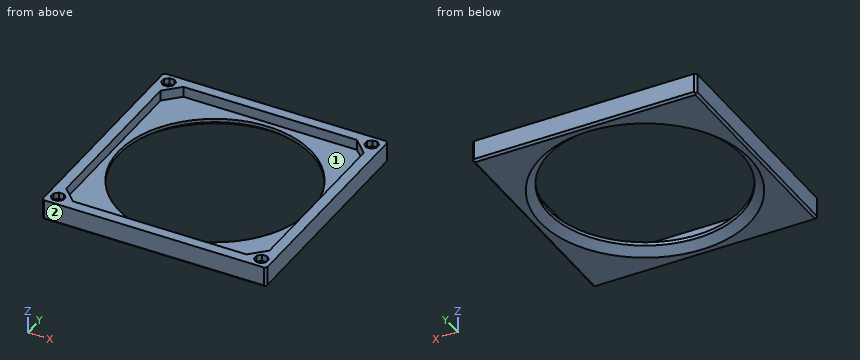
```python
from build123d import *

# Parameters (mm, degrees)
SKETCH1_LARGER_DIA_W    = 106
SKETCH1_LARGER_DIA_H    = 106
BOSS_EXTRUDE1_DEPTH     = 5
SKETCH5_SMALLER_DIA_W   = 106
SKETCH5_SMALLER_DIA_H   = 106
SKETCH5_SMALLER_DIA_R   = 45.5
BOSS_EXTRUDE2_DEPTH     = 5
CUT_EXTRUDE1_DEPTH      = 3
CHAMFER1_SIZE           = 4
CHAMFER1_SIZE2          = 3.356398525
CHAMFER2_SIZE           = 1
CHAMFER3_SIZE           = 1
CUT_EXTRUDE2_DEPTH      = 10
CUT_EXTRUDE2_DEPTH_BACK = 2
SKETCH3_HOLES_R         = 1.6


with BuildPart() as part:
    # Sketch1 larger dia → Boss-Extrude1 (new body)
    with BuildSketch(Plane.XY):
        Rectangle(SKETCH1_LARGER_DIA_W, SKETCH1_LARGER_DIA_H)
        Polygon((-41, 48), (41, 48), (48, 41), (48, -41), (41, -48), (-41, -48), (-48, -41), (-48, 41), align=None, mode=Mode.SUBTRACT)
    extrude(amount=BOSS_EXTRUDE1_DEPTH)

    # Sketch5 smaller dia → Boss-Extrude2 (add)
    with BuildSketch(Plane(origin=(0, 0, 0), x_dir=(-1, 0, 0), z_dir=(0, 0, -1))):
        Rectangle(SKETCH5_SMALLER_DIA_W, SKETCH5_SMALLER_DIA_H)
        Circle(SKETCH5_SMALLER_DIA_R, mode=Mode.SUBTRACT)
    extrude(amount=BOSS_EXTRUDE2_DEPTH)

    # Sketch1 → Cut-Extrude1 (cut)
    with BuildSketch(Plane.XY.offset(5)):
        Polygon((-45.1, 46.798780669), (-45.1, 49.201219331), (-46.798780669, 50.9), (-49.201219331, 50.9), (-50.9, 49.201219331), (-50.9, 46.798780669), (-49.201219331, 45.1), (-46.798780669, 45.1), align=None)
        Polygon((-46.798780669, -45.1), (-45.1, -46.798780669), (-45.1, -49.201219331), (-46.798780669, -50.9), (-49.201219331, -50.9), (-50.9, -49.201219331), (-50.9, -46.798780669), (-49.201219331, -45.1), align=None)
        Polygon((46.798780669, 45.1), (45.1, 46.798780669), (45.1, 49.201219331), (46.798780669, 50.9), (49.201219331, 50.9), (50.9, 49.201219331), (50.9, 46.798780669), (49.201219331, 45.1), align=None)
        Polygon((45.1, -46.798780669), (45.1, -49.201219331), (46.798780669, -50.9), (49.201219331, -50.9), (50.9, -49.201219331), (50.9, -46.798780669), (49.201219331, -45.1), (46.798780669, -45.1), align=None)
    extrude(amount=-CUT_EXTRUDE1_DEPTH, mode=Mode.SUBTRACT)

    # Chamfer1
    chamfer1_edges = [part.edges().sort_by_distance(p)[0] for p in [
        (45.5, 0, -5),
    ]]
    chamfer1_side = [part.faces().sort_by_distance(p)[0] for p in [
        (0, 51.500933624, -5),
    ]]
    chamfer(chamfer1_edges, length=CHAMFER1_SIZE, length2=CHAMFER1_SIZE2, reference=chamfer1_side[0])

    # Chamfer2
    chamfer2_edges = [part.edges().sort_by_distance(p)[0] for p in [
        (53, 0, -5),
        (0, -53, -5),
        (-53, 0, -5),
        (0, 53, -5),
    ]]
    chamfer(chamfer2_edges, length=CHAMFER2_SIZE)

    # Chamfer3
    chamfer3_edges = [part.edges().sort_by_distance(p)[0] for p in [
        (-53, 53, 0.5),
        (53, 53, 0.5),
        (53, -53, 0.5),
        (-53, -53, 0.5),
    ]]
    chamfer(chamfer3_edges, length=CHAMFER3_SIZE)

    # Sketch3 holes → Cut-Extrude2 (cut, two sides: drawn at the far end of the back side and taken through both)
    with BuildSketch(Plane.XY.offset(-CUT_EXTRUDE2_DEPTH_BACK)):
        with Locations((-48, 48)):
            Circle(SKETCH3_HOLES_R)
        with Locations(Location((48, 48, 0), (0, 0, 180))):
            Circle(SKETCH3_HOLES_R)
        with Locations(Location((-48, -48, 0), (0, 0, 180))):
            Circle(SKETCH3_HOLES_R)
        with Locations((48, -48)):
            Circle(SKETCH3_HOLES_R)
    extrude(amount=CUT_EXTRUDE2_DEPTH + CUT_EXTRUDE2_DEPTH_BACK, mode=Mode.SUBTRACT)


solid = part.part
```
Verification items for the finished model (mm, model axes). Face numbers are marked on the shaded views. Give positions to 0.01 mm unless a question says otherwise; leave off trailing zeros. Order: outer loops, then holes, each group sorted by start corner. A loop starts at its lowest first (then second) coordinate and runs counter-clockwise, first axis right, second up. Notation, with made-up numbers: (-13, -17.5) -> (5, -17.5) arc R15 ccw to (5, -12.5) -> close; hole circle Ø11 at (-38.5, -29). An arc over 180 degrees is marked (long way). One line per item, written item: value.
(1) Scan lines: line 1 along X through (y, z) = (-48, -1.2); line 2 along Y through (x, z) = (0, -0.8). Record each from-to range of solid material in increasing order. Write a range as [from, to].
Final values:
line 1: [-53, -49.6], [-46.4, 46.4], [49.6, 53]
line 2: [-53, -45.5], [45.5, 53]
(2) Sectioned sample at A-A on y = 0. Record the cut outline in (x, z).
Final values:
outline: (-53, -4) -> (-52, -5) -> (-49.5, -5) -> (-45.5, -1.64) -> (-45.5, 0) -> (-48, 0) -> (-48, 5) -> (-53, 5) -> close; (45.5, -1.64) -> (49.5, -5) -> (52, -5) -> (53, -4) -> (53, 5) -> (48, 5) -> (48, 0) -> (45.5, 0) -> close
(3) Gauge pin test, flat ends, axial feed: pin 1 (2.5 mm diameter, centred on x = 48, y = -48, fed in from +Z); pin 2 (4.5 mm diameter, centred on x = 47.5, y = -48, fed in from +Z). Record the tip position at first contact, or that the pin passes through.
Final values:
pin 1: z = -2
pin 2: z = 2
(4) Draft check along X on the marked faces 1 and 2. Enter one of: pulls with the +X half, pulls with the -X half, needs draft (parallel to the pull), parting line crosses it, or undercut.
Final values:
face 1: undercut
face 2: needs draft
